Geometry check sheet. Reference: the model listing, model coordinates, mm. Give positions to 0.01 mm unless a question says otherwise; leave off trailing zeros. Loops run counter-clockwise (first coordinate to the right, second up) from the corner with the lowest first, then second, coordinate; pieces in that order, holes last. Notation, with made-up numbers: (-5.5, 20) -> (3.5, 20) arc R22 cw to (3.5, 27) -> close; hole circle Ø8 at (42.25, 67.5). An arc over 180 degrees is marked (long way). Write item = value, one per line.
```python
from build123d import *

# Parameters (mm, degrees)
F1_DEPTH = 2.38125
F2_R     = 1.2446
F2_R_2   = 4.7625
F2_R_3   = 3.571875
F2_R_4   = 2.778125
F3_DEPTH = 2.38125


with BuildPart() as f1:
    # F0 (on Front) → F1 (new body)
    with BuildSketch(Plane.XZ):
        Polygon((282.359224, 19.05), (-44.665776, 19.05), (-44.665776, 0), (-14.503276, -33.402232), (44.234224, -47.625), (56.934224, -47.625), (56.934224, -15.875), (75.984224, -15.875), (75.984224, -47.625), (164.884224, -47.625), (164.884224, -15.875), (183.934224, -15.875), (183.934224, -47.625), (206.159224, -47.625), (282.359224, 0), align=None)
    extrude(amount=F1_DEPTH)

    # F2 (on face) → F3 (cut)
    with BuildSketch(Plane.XZ.offset(2.38125)):
        with Locations((276.009224, 11.1125)):
            Circle(F2_R)
        with Locations((276.009224, 3.175)):
            Circle(F2_R)
        with Locations((269.659224, 7.14375)):
            Circle(F2_R)
        with Locations((74.396724, 12.7)):
            Circle(F2_R_2)
        with Locations((95.034224, -17.866384)):
            Circle(F2_R)
        with Locations((95.034224, -28.978884)):
            Circle(F2_R)
        with Locations((95.034224, -40.091384)):
            Circle(F2_R)
        with Locations((-38.315776, 11.1125)):
            Circle(F2_R)
        with Locations((-38.315776, 3.175)):
            Circle(F2_R)
        with Locations((-31.965776, 7.14375)):
            Circle(F2_R)
        with BuildLine():
            ThreePointArc((21.238677, -20.095719), (22.385265, -21.431157), (23.720703, -20.284569))
            Line((23.720703, -20.284569), (21.238677, -20.095719))
        make_face()
        with BuildLine():
            ThreePointArc((-10.925388, 1.112718), (-12.260826, -0.03387), (-11.114238, -1.369308))
            Line((-11.114238, -1.369308), (-10.925388, 1.112718))
        make_face()
        with BuildLine():
            Line((-10.925388, 1.112718), (-11.114238, -1.369308))
            ThreePointArc((-11.114238, -1.369308), (-10.173791, -1.041134), (-9.775213, -0.128295))
            ThreePointArc((-9.775213, -0.128295), (-10.106974, 0.717728), (-10.925388, 1.112718))
        make_face()
        with BuildLine():
            ThreePointArc((-13.585665, -17.446041), (-12.439077, -18.781479), (-11.103639, -17.634891))
            Line((-11.103639, -17.634891), (-12.344652, -17.540466))
            Line((-12.344652, -17.540466), (-13.585665, -17.446041))
        make_face()
        with BuildLine():
            Line((-12.344652, -17.540466), (-11.103639, -17.634891))
            ThreePointArc((-11.103639, -17.634891), (-11.100949, -17.587712), (-11.100052, -17.540466))
            ThreePointArc((-11.100052, -17.540466), (-11.431813, -16.694444), (-12.250227, -16.299453))
            Line((-12.250227, -16.299453), (-12.344652, -17.540466))
        make_face()
        with BuildLine():
            ThreePointArc((3.826506, -18.77088), (4.973094, -20.106318), (6.308532, -18.95973))
            Line((6.308532, -18.95973), (3.826506, -18.77088))
        make_face()
        with BuildLine():
            Line((3.826506, -18.77088), (6.308532, -18.95973))
            ThreePointArc((6.308532, -18.95973), (6.311222, -18.912552), (6.312119, -18.865305))
            ThreePointArc((6.312119, -18.865305), (5.114765, -17.621602), (3.826506, -18.77088))
        make_face()
        with BuildLine():
            Line((21.238677, -20.095719), (23.720703, -20.284569))
            ThreePointArc((23.720703, -20.284569), (23.723393, -20.237391), (23.72429, -20.190144))
            ThreePointArc((23.72429, -20.190144), (22.526937, -18.946441), (21.238677, -20.095719))
        make_face()
        with BuildLine():
            Line((-13.585665, -17.446041), (-12.344652, -17.540466))
            Line((-12.344652, -17.540466), (-12.250227, -16.299453))
            ThreePointArc((-12.250227, -16.299453), (-13.155413, -16.596169), (-13.585665, -17.446041))
        make_face()
        with Locations((23.804529, -2.777973)):
            Circle(F2_R)
        with Locations((6.392358, -1.453134)):
            Circle(F2_R_3)
        with Locations((-2.287686, 11.944013)):
            Circle(F2_R_4)
    extrude(amount=-F3_DEPTH, mode=Mode.SUBTRACT)


solid = f1.part
```
Item 1: Section check A-A, the plane z = -25. Record the cut outline in (x, y), plus the area to 3 significant figures.
Answer:
outline = (-22.09, -2.38) -> (56.93, -2.38) -> (56.93, 0) -> (-22.09, 0) -> close; (75.98, -2.38) -> (164.88, -2.38) -> (164.88, 0) -> (75.98, 0) -> close; (183.93, -2.38) -> (242.36, -2.38) -> (242.36, 0) -> (183.93, 0) -> close
area = 539 mm^2
Item 2: Draft check along X on faces 1 (the flat face through (-29.796, -1.174, -16.467)), 2 (the flat face through (117, 0, -14)), 3 (the cylindrical face through (-2.65, -1.21, 14.7)). Enter one of: +X half, -X half, draft (parallel to the pull), parting line (faces both ways), or undercut.
Answer:
face_1 = -X half
face_2 = draft
face_3 = undercut
Item 3: Section check B-B, the plane y = -1.75. Give the number of separate pieces and of enclosed holes in the cut face, plus the area to 3 significant figures.
Answer:
separate_pieces = 1
enclosed_holes = 17
area = 17,200 mm^2
Item 4: Thickness scan on L1, parallel to X at y = -0.5, z = -16; L2, parallel to X at y = -0.35, z = -2.5; L3, parallel to X at y = -0.4, z = -16.5. Record the ranges inside material, lowest first. Write a range as [from, to].
Answer:
L1 = [-30.22, 56.93], [75.98, 164.88], [183.93, 256.76]
L2 = [-42.41, 2.98], [9.81, 22.59], [25.02, 278.36]
L3 = [-29.77, -13.03], [-11.66, 56.93], [75.98, 164.88], [183.93, 255.96]
Item 5: Section check D-D, the plane z = -10.5. Record the cut outline in (x, y).
Answer:
outline = (-35.18, -2.38) -> (265.56, -2.38) -> (265.56, 0) -> (-35.18, 0) -> close
Item 6: Gauge pin test, flat ends, axial feed: pin 1 (2 mm diameter, centred on x = 8, z = 4, fed in from +Y); pin 2 (1.5 mm diameter, centred on x = 276.01, z = 11.11, fed in from +Y); pin 3 (1.2 mm diameter, centred on x = 172, y = -1.5, fed in from -Z) (3 decimals). Record the tip position at first contact, or that the pin passes through.
Answer:
pin_1 = 0
pin_2 = through
pin_3 = -15.875
Item 7: Section check C-C, the plane x = 256. Record the cut outline in (y, z), plus the area to 3 significant figures.
Answer:
outline = (-2.38, -16.47) -> (0, -16.47) -> (0, 19.05) -> (-2.38, 19.05) -> close
area = 84.6 mm^2
